from build123d import *

# Parameters (mm, degrees)
F1_DEPTH      = 25.4
F2_DEPTH      = 25.4
F3_DEPTH      = 25.4
F4_DEPTH      = 25.4
F6_R          = 21.9155867699
F6_R_2        = 16.2549330377
F7_DEPTH      = 25.4
F7_DEPTH_BACK = 25.4


with BuildPart() as f1:
    # F0 (on Right) → F1 (new body)
    with BuildSketch(Plane.YZ):
        Polygon((-50.3195412457, 0), (0, 0), (46.4636348188, 0), (46.4636348188, 19.8579039425), (29.1120689362, 19.8579039425), (29.1120689362, 35.6671102345), (-27.955301106, 35.6671102345), (-27.955301106, 19.8579039425), (-50.3195412457, 19.8579039425), align=None)
    extrude(amount=F1_DEPTH)

    # F2 (add): a face of the model
    f2_faces = [f1.faces().sort_by_distance(p)[0] for p in [
        (25.4, -1.1272764722, 15.6260757274),
    ]]
    extrude(f2_faces, amount=F2_DEPTH)

    # F3 (add): a face of the model
    f3_faces = [f1.faces().sort_by_distance(p)[0] for p in [
        (50.8, -1.1272764722, 15.6260757274),
    ]]
    extrude(f3_faces, amount=F3_DEPTH)

    # F4 (add): a face of the model
    f4_faces = [f1.faces().sort_by_distance(p)[0] for p in [
        (76.2, -1.1272764722, 15.6260757274),
    ]]
    extrude(f4_faces, amount=F4_DEPTH)

    # F6 (on face) → F7 (join, two sides)
    with BuildSketch(Plane.XY.offset(35.6671102345)) as f7_sk:
        with Locations((49.8246699572, 0)):
            Circle(F6_R)
        with Locations((49.8246699572, 0)):
            Circle(F6_R_2, mode=Mode.SUBTRACT)
    extrude(amount=F7_DEPTH)
    extrude(f7_sk.sketch, amount=-F7_DEPTH_BACK)


solid = f1.part
CAD build for the part. Positions are in the model's coordinates, mm. A direction names the side the tool comes from. Round coordinates to 2 decimals unless told otherwise and drop trailing zeros. Loops run counter-clockwise (first coordinate to the right, second up) from the corner with the lowest first, then second, coordinate; pieces in that order, holes last. Notation, with made-up numbers: M 74.25,-15 L 122.25,-15 A29 cw 122.25,6 Z; hole C 20.5,20 d3. An arc over 180 degrees is marked long. One line per question, with ' | ' between items. Start each with the question number.
Item 1: Pin check, flat tips, straight feed: pin 1 Ø12.5 at (x, z) = (63.5, 25.5) entering from +Y; pin 2 Ø4 at (x, y) = (19.5, 24.5) entering from +Z; pin 3 Ø3 at (x, z) = (52, 29.5) entering from -Y; pin 4 Ø11 at (x, y) = (45.5, -34) entering from +Z. Stop position of each tip, or through.
Item 2: Cut at A-A, the plane x = 11. Write the cut outline in (y, z).
Item 3: Cut at C-C, the plane z = 53. Write the cut outline in (x, y).
Item 4: Wall check: line 1 (Y direction, x = 76, z = 24.5); line 2 (Z direction, x = 6.5, y = -7); line 3 (Z direction, x = 30, y = -39.5). Give the ranges that are in metal, low to high.
Item 5: Cut at B-B, the plane y = 0. Write the cut outline in (x, z).
Item 6: Which spindle directions (+Z, -Z, +X, -X, +Y, -Y) get a long thin tool onto all of the face, cutting with end or side? Do faces 1 (the flat face through (50, 38, 19.858)), 2 (the flat face through (50, -39, 19.858)), 3 (the cylindrical face through (70.73, 6.58, 48.19)). Say none if no direction does.
Item 7: Two-plate mould, pull along Y, no slides. Class faces 4 (the flat face through (50, 29.112, 28)), 5 (the cylindrical face through (65.33, 4.88, 48.19)), 6 (the flat face through (101.6, -3, 14)): pulls with the +Y half, pulls with the -Y half, needs draft (parallel to the pull), parting line crosses it, or undercut.
Item 8: Cut at D-D, the plane z = 26. Write the cut outline in (x, y).
Responses:
1) pin 1: stops at y = 46.46 | pin 2: stops at z = 35.67 | pin 3: stops at y = -27.96 | pin 4: stops at z = 19.86
2) outline: M -50.32,0 L 46.46,0 L 46.46,19.86 L 29.11,19.86 L 29.11,35.67 L -27.96,35.67 L -27.96,19.86 L -50.32,19.86 Z
3) outline: C 49.82,0 d43.83; hole C 49.82,0 d32.51
4) line 1: y = -27.96 to 29.11 | line 2: z = 0 to 35.67 | line 3: z = 0 to 19.86
5) outline: M 0,0 L 101.6,0 L 101.6,35.67 L 71.74,35.67 L 71.74,61.07 L 66.08,61.07 L 66.08,35.67 L 33.57,35.67 L 33.57,61.07 L 27.91,61.07 L 27.91,35.67 L 0,35.67 Z
6) face 1: +Z, +X, -X, +Y | face 2: +Z, +X, -X, -Y | face 3: +Z
7) face 4: pulls with the +Y half | face 5: undercut | face 6: needs draft
8) outline: M 0,-27.96 L 101.6,-27.96 L 101.6,29.11 L 0,29.11 Z
